The model under review builds one solid part; all positions refer to its coordinate system, in mm. Face numbers are marked on the shaded views. A direction names the side the tool comes from. Round coordinates to 2 decimals unless told otherwise and drop trailing zeros. Write each loop counter-clockwise with the first axis right and the second up, starting at its lowest first coordinate (ties: lowest second). Pieces come first, ordered by that corner, then holes.
Item 1: Add section C-C (y = 13.5). Give the boundary of the cut face in (x, z) (3 decimals).
Item 2: Machinability: for the marked faces 5 and 6, which of the approach directions +Z, -Z, +X, -X, +Y, -Y give a long, thin tool a straight path to every point of the face, cutting with its end or side? Answer none if there is none.
Item 3: To check wall thickness, follow L1, parallel to X at y = 1.5, z = -10; L2, parallel to X at y = 6.25, z = 11; L3, parallel to X at y = 3.5, z = -19. State the ranges of each line that lie inside material, in increasing order.
Item 4: Add section B-B (z = 16.51). Give the boundary of the cut face in (x, y) (3 decimals), plus the area to 3 significant figures.
Item 5: Draft analysis for pull direction Z (two halves, no side actions). For the marked faces 1, 2, 3 and 4, state which applies: +Z half, -Z half, draft (parallel to the pull), parting line (faces both ways), or undercut.
Item 6: Clearance check with flat-ended pins moving along their axes: pin 1 Ø3 at (x, z) = (-1, -16) entering from -Y; pin 2 Ø1 at (x, y) = (-16, 8.5) entering from -Z; pin 3 Ø10 at (y, z) = (7.5, 16) entering from -X; pin 4 Ø2 at (x, z) = (14.5, -8.5) entering from -Y. State where each tip first meets the part, or that it passes through.
```python
from build123d import *
from OCP.BRepFilletAPI import BRepFilletAPI_MakeChamfer

# Parameters (mm, degrees)
SKETCH2_R                     = 27
BOSS_EXTRUDE2_DEPTH           = 20
CBORE_FOR_M3_SHCS1_AT_2_COUNT = 2
CBORE_FOR_M3_SHCS1_AT_2_PITCH = 28.596158833
CBORE_FOR_M3_SHCS1_AT_3_COUNT = 2
CBORE_FOR_M3_SHCS1_AT_3_PITCH = 28.596158833
HOLE1_D                       = 6.4
HOLE1_DEPTH                   = 15
HOLE1_CBORE_D                 = 7.3
HOLE1_CBORE_DEPTH             = 2
CHAMFER1_SIZE                 = 2
CHAMFER1_SIZE_2               = 0.45


with BuildPart() as part:
    # Sketch2 → Boss-Extrude2 (new body)
    with BuildSketch(Plane(origin=(0, 0, 0), x_dir=(1, 0, 0), z_dir=(0, 1, 0))):
        with Locations(Location((0, 0, 0), (0, 0, 270))):
            Circle(SKETCH2_R)
    extrude(amount=BOSS_EXTRUDE2_DEPTH)

    # Sketch5 → CBORE for M3 SHCS1 (revolve, cut)
    with BuildSketch(Plane(origin=(0, 0, 16.51), x_dir=(0, 0, -1), z_dir=(1, 0, 0))):
        Polygon((0, 0), (0, 20), (1.8, 20), (1.8, 16), (3.25, 16), (3.25, 0.025), (3.275, 0), align=None)
    cbore_for_m3_shcs1 = revolve(axis=Axis((0, -6.35, 16.51), (0, 1, 0)), mode=Mode.SUBTRACT)

    # CBORE for M3 SHCS1 at 2: CBORE for M3 SHCS1 ×2
    with Locations(*[Vector(0.5000000000000012, 0, -0.8660254037844379) * (i * CBORE_FOR_M3_SHCS1_AT_2_PITCH) for i in range(1, CBORE_FOR_M3_SHCS1_AT_2_COUNT)]):
        add(cbore_for_m3_shcs1, mode=Mode.SUBTRACT)

    # CBORE for M3 SHCS1 at 3: CBORE for M3 SHCS1 ×2
    with Locations(*[Vector(-0.4999999999999978, 0, -0.8660254037844399) * (i * CBORE_FOR_M3_SHCS1_AT_3_PITCH) for i in range(1, CBORE_FOR_M3_SHCS1_AT_3_COUNT)]):
        add(cbore_for_m3_shcs1, mode=Mode.SUBTRACT)

    # Hole1
    with Locations(Plane(origin=(0, 0, 0), x_dir=(-1, 0, 0), z_dir=(0, -1, 0))):
        with Locations((14.298079416, -8.255), (0, 16.51), (-14.298079416, -8.255)):
            CounterBoreHole(HOLE1_D / 2, HOLE1_CBORE_D / 2, HOLE1_CBORE_DEPTH, depth=HOLE1_DEPTH)

    # Chamfer1
    chamfer1_edges_1 = [part.edges().sort_by_distance(p)[0] for p in [
        (17.948079416, 2, 8.255),
    ]]
    chamfer1_side_1 = [part.faces().sort_by_distance(p)[0] for p in [
        (17.948079416, 1.991, 8.255),
    ]]
    chamfer1_edges_2 = [part.edges().sort_by_distance(p)[0] for p in [
        (3.65, 2, -16.51),
    ]]
    chamfer1_side_2 = [part.faces().sort_by_distance(p)[0] for p in [
        (3.65, 1.991, -16.51),
    ]]
    chamfer1_edges_3 = [part.edges().sort_by_distance(p)[0] for p in [
        (-10.648079416, 2, 8.255),
    ]]
    chamfer1_side_3 = [part.faces().sort_by_distance(p)[0] for p in [
        (-10.648079416, 1.991, 8.255),
    ]]
    chamfer1 = BRepFilletAPI_MakeChamfer(part.part.solid().wrapped)
    for e in chamfer1_edges_1:
        chamfer1.Add(CHAMFER1_SIZE - 0.0001, CHAMFER1_SIZE_2 - 0.0001, e.wrapped, chamfer1_side_1[0].wrapped)
    for e in chamfer1_edges_2:
        chamfer1.Add(CHAMFER1_SIZE - 0.0001, CHAMFER1_SIZE_2 - 0.0001, e.wrapped, chamfer1_side_2[0].wrapped)
    for e in chamfer1_edges_3:
        chamfer1.Add(CHAMFER1_SIZE - 0.0001, CHAMFER1_SIZE_2 - 0.0001, e.wrapped, chamfer1_side_3[0].wrapped)
    add(Compound.cast(chamfer1.Shape()), mode=Mode.REPLACE)  # a hair under: the kernel refuses the full size


solid = part.part
```
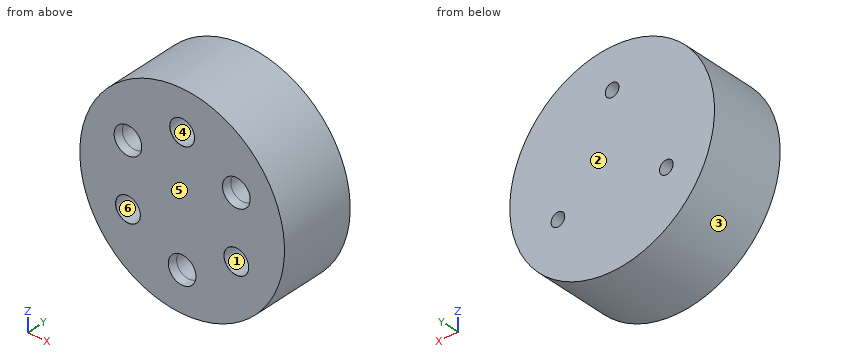
Numbers:
1. outline: circle Ø54 at (0, 0); hole circle Ø6.5 at (-14.298, -8.255); hole circle Ø6.4 at (-14.298, 8.255); hole circle Ø6.5 at (0, 16.51); hole circle Ø6.4 at (0, -16.51); hole circle Ø6.5 at (14.298, -8.255); hole circle Ø6.4 at (14.298, 8.255)
2. face 5: +Z, -Z, +X, -X, -Y
2. face 6: -Y
3. L1: x = -25.08 to -17.04, -11.56 to 11.56, 17.04 to 25.08
3. L2: x = -24.66 to -15.94, -12.65 to 12.65, 15.94 to 24.66
3. L3: x = -19.18 to -2.01, 2.01 to 19.18
4. outline: (-21.364, 0) - (-3.275, 0) - (-3.25, 0.025) - (-3.25, 16) - (-1.8, 16) - (-1.8, 20) - (-21.364, 20) - close; (1.8, 16) - (3.25, 16) - (3.25, 0.025) - (3.275, 0) - (21.364, 0) - (21.364, 20) - (1.8, 20) - close
4. area: 736 mm2
5. face 1: undercut
5. face 2: draft
5. face 3: parting line
5. face 4: undercut
6. pin 1: stops at y = 15
6. pin 2: stops at z = -22.11
6. pin 3: stops at x = -24.66
6. pin 4: passes through
